from build123d import *

# Parameters (mm, degrees)
PAD_DEPTH             = 24
POCKET_DEPTH          = 3
SKETCH002_W           = 70
SKETCH002_H           = 18.5
POCKET001_DEPTH       = 18
POLARPATTERN_COUNT    = 3
POCKET002_DEPTH       = 6
CHAMFER_SIZE          = 8
FILLET_R              = 13
FILLET001_R           = 11
CHAMFER001_SIZE       = 16.1
FILLET002_R           = 11
FILLET003_R           = 12
POCKET003_DEPTH       = 6
POCKET004_DEPTH       = 18
POCKET005_DEPTH       = 21.001
SKETCH012_R           = 1.85
SKETCH012_R_2         = 0.99
POCKET011_DEPTH       = 498.049286
POLARPATTERN001_COUNT = 3


with BuildPart() as part:
    # Sketch → Pad (new body)
    with BuildSketch(Plane.XY):
        Polygon((0, 112.209492), (-97.17627, -56.104746), (97.17627, -56.104746), align=None)
        Polygon((0, 62.209492), (-53.875, -31.104746), (53.875, -31.104746), align=None, mode=Mode.SUBTRACT)
    extrude(amount=PAD_DEPTH)

    # Sketch001 (on Face8 of Pad) → Pocket (cut)
    with BuildSketch(Plane.XY.offset(24)):
        Polygon((0, 98.209492), (-85.051915, -49.104746), (85.051915, -49.104746), align=None)
        Polygon((0, 76.209492), (-65.999356, -38.104746), (65.999356, -38.104746), align=None, mode=Mode.SUBTRACT)
    extrude(amount=-POCKET_DEPTH, mode=Mode.SUBTRACT)

    # Sketch002 (on Face4 of Pocket) → Pocket001 (cut)
    with BuildSketch(Plane(origin=(0, 0, 0), x_dir=(1, 0, 0), z_dir=(0, 0, -1))):
        with Locations((0, 43.604746)):
            Rectangle(SKETCH002_W, SKETCH002_H)
    pocket001 = extrude(amount=-POCKET001_DEPTH, mode=Mode.SUBTRACT)

    # PolarPattern: Pocket001 ×3 about axis
    polarpattern_axis = Axis((0, 0, 0), (0, 0, -1))
    for i in range(1, POLARPATTERN_COUNT):
        add(pocket001.rotate(polarpattern_axis, i * 360 / POLARPATTERN_COUNT), mode=Mode.SUBTRACT)

    # Sketch003 (on Face4 of PolarPattern) → Pocket002 (cut)
    with BuildSketch(Plane(origin=(0, 0, 0), x_dir=(1, 0, 0), z_dir=(0, 0, -1))):
        Polygon((0, -100.209492), (86.783965, 50.104746), (-86.783965, 50.104746), align=None)
        Polygon((0, -74.209492), (64.267305, 37.104746), (-64.267305, 37.104746), align=None, mode=Mode.SUBTRACT)
    extrude(amount=-POCKET002_DEPTH, mode=Mode.SUBTRACT)

    # Chamfer
    chamfer_edges = [part.edges().sort_by_distance(p)[0] for p in [
        (-53.875, -31.104746, 12),
        (53.875, -31.104746, 12),
        (0, 62.209492, 12),
    ]]
    chamfer(chamfer_edges, length=CHAMFER_SIZE)

    # Fillet
    fillet_edges = [part.edges().sort_by_distance(p)[0] for p in [
        (0, 100.209492, 3),
        (-86.783965, -50.104746, 3),
        (86.783965, -50.104746, 3),
    ]]
    fillet(fillet_edges, radius=FILLET_R)

    # Fillet001
    fillet001_edges = [part.edges().sort_by_distance(p)[0] for p in [
        (0, 74.209492, 3),
        (64.267305, -37.104746, 3),
        (-64.267305, -37.104746, 3),
    ]]
    fillet(fillet001_edges, radius=FILLET001_R)

    # Chamfer001
    chamfer001_edges = [part.edges().sort_by_distance(p)[0] for p in [
        (97.17627, -56.104746, 12),
        (0, 112.209492, 12),
        (-97.17627, -56.104746, 12),
    ]]
    chamfer(chamfer001_edges, length=CHAMFER001_SIZE)

    # Fillet002
    fillet002_edges = [part.edges().sort_by_distance(p)[0] for p in [
        (0, 98.209492, 22.5),
        (-85.051915, -49.104746, 22.5),
        (85.051915, -49.104746, 22.5),
    ]]
    fillet(fillet002_edges, radius=FILLET002_R)

    # Fillet003
    fillet003_edges = [part.edges().sort_by_distance(p)[0] for p in [
        (65.999356, -38.104746, 22.5),
        (0, 76.209492, 22.5),
        (-65.999356, -38.104746, 22.5),
    ]]
    fillet(fillet003_edges, radius=FILLET003_R)

    # Sketch004 (on Face60 of Fillet003) → Pocket003 (cut)
    with BuildSketch(Plane(origin=(0, 0, 6), x_dir=(1, 0, 0), z_dir=(0, 0, -1))):
        Polygon((-8.75, -71.266483), (8.75, -71.266483), (8.75, -94.766483), (4, -94.766483), (4, -98.266483), (-4, -98.266483), (-4, -94.766483), (-8.75, -94.766483), align=None)
    extrude(amount=-POCKET003_DEPTH, mode=Mode.SUBTRACT)

    # Sketch005 (on Face29 of Pocket003) → Pocket004 (cut)
    with BuildSketch(Plane(origin=(0, 0, 0), x_dir=(1, 0, 0), z_dir=(0, 0, -1))):
        Polygon((46.171599, 38.954746), (68.688259, 51.954746), (79.338259, 33.508405), (56.821599, 20.508405), align=None)
    extrude(amount=-POCKET004_DEPTH, mode=Mode.SUBTRACT)

    # Sketch006 (on Face1 of Pocket004) → Pocket005 (cut, through all)
    with BuildSketch(Plane.XY.offset(21)):
        with BuildLine():
            ThreePointArc((1.5, 85.040452), (0, 86.540452), (-1.5, 85.040452))
            Line((-1.5, 85.040452), (-1.5, 66.040452))
            ThreePointArc((-1.5, 66.040452), (0, 64.540452), (1.5, 66.040452))
            Line((1.5, 85.040452), (1.5, 66.040452))
        make_face()
    extrude(amount=-POCKET005_DEPTH, mode=Mode.SUBTRACT)

    # Sketch012 → Pocket011 (cut, through all)
    with BuildSketch(Plane(origin=(0, 0, 0), x_dir=(1, 0, 0), z_dir=(0, 0, -1))):
        with Locations((-13.5, -82.703211)):
            Circle(SKETCH012_R)
        with Locations((13.5, -82.703211)):
            Circle(SKETCH012_R)
        with Locations((-6.25, -96.516483)):
            Circle(SKETCH012_R_2)
        with Locations((6.25, -96.516483)):
            Circle(SKETCH012_R_2)
        with Locations((-27.246325, -59.017473)):
            Circle(SKETCH012_R_2)
        with Locations((-47.186207, -27.240583)):
            Circle(SKETCH012_R_2)
        with Locations((-64.733793, 5.912727)):
            Circle(SKETCH012_R_2)
        with Locations((-10.791842, -49.517473)):
            Circle(SKETCH012_R_2)
        with Locations((-28.339428, -16.364163)):
            Circle(SKETCH012_R_2)
        with Locations((-48.279311, 15.412727)):
            Circle(SKETCH012_R_2)
    pocket011 = extrude(amount=-POCKET011_DEPTH, mode=Mode.SUBTRACT)

    # PolarPattern001: Pocket011 ×3 about axis
    polarpattern001_axis = Axis((0, 0, 0), (0, 0, -1))
    for i in range(1, POLARPATTERN001_COUNT):
        add(pocket011.rotate(polarpattern001_axis, i * 360 / POLARPATTERN001_COUNT), mode=Mode.SUBTRACT)


solid = part.part
Work out the finished part from the listing and answer in its coordinate system (mm). A direction names the side the tool comes from. Coordinates: 2 decimals unless noted, no trailing zeros.
1. For faces 3 (the cylindrical face through (66.58, -52.33, 11.83)), 4 (the flat face through (0, -41, 21)), 5 (the cylindrical face through (-0.16, 63.21, 3.04)), determine the directions among +Z, -Z, +X, -X, +Y, -Y from which every point of the face is accessible in a straight line to the end or side of a thin tool.
Results list:
face 3: +Z, -Z
face 4: +Z
face 5: -Z
2. Flat-ended cylindrical pins translate along their axes: pin 1 (1.5 mm diameter, centred on x = 65.5, y = -17.5, fed in from -Z); pin 2 (5.5 mm diameter, centred on y = -46.5, z = 5, fed in from -X); pin 3 (6 mm diameter, centred on y = 48, z = 15, fed in from -X); pin 4 (2 mm diameter, centred on x = 78.37, y = -29.66, fed in from -Z). Find the tip coordinate at first contact, or state that the pin passes through.
Results list:
pin 1: stops at z = 6
pin 2: stops at x = -88.21
pin 3: stops at x = -38.8
pin 4: passes through
3. The part is cut by section A-A, the plane z = 15.25. State how many separate pieces and enclosed holes the cut face has, and give its area (3 significant figures).
Results list:
separate pieces: 1
enclosed holes: 36
area: 6,430 mm2
4. For a pull along Y with two mould halves and no side action, classify faces 1 (the flat face through (-1, -56.105, 12)), 2 (the cylindrical face through (-12.646, 84.344, 11.832)) as +Y half, -Y half, draft (parallel to the pull), parting line (faces both ways), or undercut.
Results list:
face 1: -Y half
face 2: undercut
5. Consider line 1 along X through (y, z) = (59, 17.5); line 2 along X through (y, z) = (84, 5.25); line 3 along X through (y, z) = (51.5, 1.75). Determine where each line is inside the solid, lowest interval first.
Results list:
line 1: x = -30.72 to -28.24, -26.26 to 26.26, 28.24 to 30.72
line 2: x = -16.29 to -14.82, -12.18 to -8.55, 8.55 to 12.18, 14.82 to 16.29
line 3: x = -35.05 to -31.3, -13.11 to -6.18, 6.18 to 13.11, 31.3 to 35.05
